Here's how the part is built. I have some questions about the finished solid (model axes, mm). Round coordinates to 2 decimals unless told otherwise and drop trailing zeros. Loops run counter-clockwise (first coordinate to the right, second up) from the corner with the lowest first, then second, coordinate; pieces in that order, holes last. Notation, with made-up numbers: M 8,-17.75 L 29,-17.75 A27 cw 29,10.25 Z; hole C 50.5,48.25 d6. An arc over 180 degrees is marked long. Use a Markdown table: item, result.
from build123d import *

# Parameters (mm, degrees)
SKETCH1_W           = 300
SKETCH1_H           = 300
BOSS_EXTRUDE1_DEPTH = 10
SKETCH2_R           = 5
CUT_EXTRUDE1_DEPTH  = 10
FILLET2_R           = 10
FILLET3_R           = 10


with BuildPart() as part:
    # Sketch1 → Boss-Extrude1 (new body)
    with BuildSketch(Plane(origin=(0, 0, 0), x_dir=(1, 0, 0), z_dir=(0, 1, 0))):
        Rectangle(SKETCH1_W, SKETCH1_H)
    extrude(amount=BOSS_EXTRUDE1_DEPTH)

    # Sketch2 → Cut-Extrude1 (cut)
    with BuildSketch(Plane(origin=(0, 10, 0), x_dir=(1, 0, 0), z_dir=(0, 1, 0))):
        with Locations(Location((-19, 80, 0), (0, 0, 270))):
            Circle(SKETCH2_R)
        with Locations(Location((19, 80, 0), (0, 0, 270))):
            Circle(SKETCH2_R)
    extrude(amount=-CUT_EXTRUDE1_DEPTH, mode=Mode.SUBTRACT)

    # Fillet2
    fillet2_edges = [part.edges().sort_by_distance(p)[0] for p in [
        (-150, 10, 0),
    ]]
    fillet(fillet2_edges, radius=FILLET2_R - 0.0001)  # a hair under: the kernel refuses the full size

    # Fillet3
    fillet3_edges = [part.edges().sort_by_distance(p)[0] for p in [
        (150, 10, 0),
    ]]
    fillet(fillet3_edges, radius=FILLET3_R - 0.0001)  # a hair under: the kernel refuses the full size


solid = part.part
1. Imagine slicing it at B-B, the plane z = -80. State how many separate pieces and enclosed holes the cut face has, then the cut area to 3 significant figures.
Answer sheet:
| item | result |
|---|---|
| separate pieces | 3 |
| enclosed holes | 0 |
| area | 2,760 mm2 |
2. I need wall thicknesses on probe 1 along X at (y, z) = (2.75, -80); probe 2 along X at (y, z) = (6, -80); probe 3 along X at (y, z) = (8.5, 70). Which ranges of each line are inside material? Lowest first, please. Write a range as from..to.
Answer sheet:
| item | result |
|---|---|
| probe 1 | -149.61..-24, -14..14, 24..149.61 |
| probe 2 | -148..-24, -14..14, 24..148 |
| probe 3 | -145.27..145.27 |
3. Imagine slicing it at A-A, the plane x = -19. Write out the boundary of the cut face in (y, z).
Answer sheet:
| item | result |
|---|---|
| outline | M 0,-150 L 10,-150 L 10,-85 L 0,-85 Z; M 0,-75 L 10,-75 L 10,150 L 0,150 Z |
4. For pin 1 Ø2 at (y, z) = (4.5, -2) entering from -X; pin 2 Ø6 at (x, z) = (19, -80) entering from +Y (3 decimals); pin 3 Ø1 at (y, z) = (3.5, 89.5) entering from -X, each with a flat end and sliding along its axis, tell me the tip position at first contact or that it passes through.
Answer sheet:
| item | result |
|---|---|
| pin 1 | x = -149.37 |
| pin 2 | through |
| pin 3 | x = -149.54 |
5. We'd pull the mould along Z, two halves only. Please class faces 1 (the face through (146.99, 7.15, -2.1)), 2 (the face through (-2, 5, 150)), 3 (the face through (17.085, 5.07, -75.381)): +Z half, -Z half, draft (parallel to the pull), parting line (faces both ways), or undercut.
Answer sheet:
| item | result |
|---|---|
| face 1 | draft |
| face 2 | +Z half |
| face 3 | undercut |
6. Imagine slicing it at C-C, the plane y = 7.25. Write out the boundary of the cut face in (x, z), then the cut area to 3 significant figures.
Answer sheet:
| item | result |
|---|---|
| outline | M -146.89,-150 L 146.89,-150 L 146.89,150 L -146.89,150 Z; hole C -19,-80 d10; hole C 19,-80 d10 |
| area | 88,000 mm2 |
